For this review, take the finished solid that the model builds, in its own axes (mm). A direction names the side the tool comes from. Coordinates: 2 decimals unless noted, no trailing zeros. Write each loop counter-clockwise with the first axis right and the second up, starting at its lowest first coordinate (ties: lowest second). Pieces come first, ordered by that corner, then holes.
```python
from build123d import *

# Parameters (mm, degrees)
F0_W      = 76.2
F0_H      = 76.2
F1_DEPTH  = 76.2
F4_DEPTH  = 76.2
F5_DEPTH  = 76.2
F8_DEPTH  = 76.2
F9_DEPTH  = 76.2
F11_DEPTH = 76.2
F13_DEPTH = 76.2
F14_DEPTH = 25.4
F15_DEPTH = 25.4
F16_DEPTH = 25.4
F17_DEPTH = 25.4
F18_DEPTH = 25.4
F19_DEPTH = 25.4
F20_DEPTH = 25.4
F21_DEPTH = 25.4
F22_DEPTH = 25.4


with BuildPart() as f1:
    # F0 (on Front) → F1 (new body)
    with BuildSketch(Plane.XZ):
        Rectangle(F0_W, F0_H)
    extrude(amount=F1_DEPTH)

    # F2 (on face) → F4 (join)
    with BuildSketch(Plane.XZ.offset(76.2)):
        with BuildLine():
            ThreePointArc((0, -38.1), (26.9407683632, -26.9407683632), (38.1, 0))
            ThreePointArc((38.1, 0), (26.9407683632, 26.9407683632), (0, 38.1))
            ThreePointArc((0, 38.1), (-26.9407683632, 26.9407683632), (-38.1, 0))
            ThreePointArc((-38.1, 0), (-26.9407683632, -26.9407683632), (0, -38.1))
        make_face()
    extrude(amount=-F4_DEPTH)

    # F3 (on face) → F5 (join)
    with BuildSketch(Plane.YZ.offset(38.1)):
        with BuildLine():
            ThreePointArc((-38.1, -38.1), (-11.1592316368, -26.9407683632), (0, 0))
            ThreePointArc((0, 0), (-11.1592316368, 26.9407683632), (-38.1, 38.1))
            ThreePointArc((-38.1, 38.1), (-65.0407683632, 26.9407683632), (-76.2, 0))
            ThreePointArc((-76.2, 0), (-65.0407683632, -26.9407683632), (-38.1, -38.1))
        make_face()
    extrude(amount=-F5_DEPTH)

    # F7 (on face) → F8 (join)
    with BuildSketch(Plane(origin=(0, 0, 0), x_dir=(-1, 0, 0), z_dir=(0, 1, 0))):
        with BuildLine():
            ThreePointArc((0, -38.1), (26.9407683632, -26.9407683632), (38.1, 0))
            ThreePointArc((38.1, 0), (26.9407683632, 26.9407683632), (0, 38.1))
            ThreePointArc((0, 38.1), (-26.9407683632, 26.9407683632), (-38.1, 0))
            ThreePointArc((-38.1, 0), (-26.9407683632, -26.9407683632), (0, -38.1))
        make_face()
    extrude(amount=-F8_DEPTH)



with BuildPart() as f9:
    # F6 (on face) → F9 (new body)
    with BuildSketch(Plane(origin=(-38.1, 0, 0), x_dir=(0, -1, 0), z_dir=(-1, 0, 0))):
        with BuildLine():
            ThreePointArc((38.1, -38.1), (65.0407683632, -26.9407683632), (76.2, 0))
            ThreePointArc((76.2, 0), (65.0407683632, 26.9407683632), (38.1, 38.1))
            ThreePointArc((38.1, 38.1), (11.1592316368, 26.9407683632), (0, 0))
            ThreePointArc((0, 0), (11.1592316368, -26.9407683632), (38.1, -38.1))
        make_face()
    extrude(amount=-F9_DEPTH)


with BuildPart() as f1_1:
    add(f1.part)

    add(f9.part)  # F11 merges F9
    # F10 (on face) → F11 (join)
    with BuildSketch(Plane.XY.offset(38.1)):
        with BuildLine():
            ThreePointArc((0, -76.2), (26.9407683632, -65.0407683632), (38.1, -38.1))
            ThreePointArc((38.1, -38.1), (26.9407683839, -11.1592316575), (5.86e-08, 0))
            ThreePointArc((5.86e-08, 0), (-26.9407683425, -11.1592316161), (-38.1, -38.1))
            ThreePointArc((-38.1, -38.1), (-26.9407683632, -65.0407683632), (0, -76.2))
        make_face()
    extrude(amount=-F11_DEPTH)

    # F12 (on face) → F13 (join)
    with BuildSketch(Plane(origin=(0, 0, -38.1), x_dir=(1, 0, 0), z_dir=(0, 0, -1))):
        with BuildLine():
            ThreePointArc((8.43e-08, 0), (26.940768393, 11.1592316666), (38.1, 38.1))
            ThreePointArc((38.1, 38.1), (26.9407683632, 65.0407683632), (0, 76.2))
            ThreePointArc((0, 76.2), (-26.9407683632, 65.0407683632), (-38.1, 38.1))
            ThreePointArc((-38.1, 38.1), (-26.9407683334, 11.159231607), (8.43e-08, 0))
        make_face()
    extrude(amount=-F13_DEPTH)

    # F2 (on face) → F14 (cut)
    with BuildSketch(Plane.XZ.offset(76.2)):
        with BuildLine():
            ThreePointArc((0, 38.1), (26.9407683632, 26.9407683632), (38.1, 0))
            Line((38.1, 0), (38.1, 38.1))
            Line((38.1, 38.1), (0, 38.1))
        make_face()
    extrude(amount=-F14_DEPTH, mode=Mode.SUBTRACT)

    # F2 (on face) → F15 (cut)
    with BuildSketch(Plane.XZ.offset(76.2)):
        with BuildLine():
            ThreePointArc((-38.1, 0), (-26.9407683632, 26.9407683632), (0, 38.1))
            Line((0, 38.1), (-38.1, 38.1))
            Line((-38.1, 38.1), (-38.1, 0))
        make_face()
    extrude(amount=-F15_DEPTH, mode=Mode.SUBTRACT)

    # F2 (on face) → F16 (cut)
    with BuildSketch(Plane.XZ.offset(76.2)):
        with BuildLine():
            Line((38.1, -38.1), (38.1, 0))
            ThreePointArc((38.1, 0), (26.9407683632, -26.9407683632), (0, -38.1))
            Line((0, -38.1), (38.1, -38.1))
        make_face()
        with BuildLine():
            Line((-38.1, -38.1), (0, -38.1))
            ThreePointArc((0, -38.1), (-26.9407683632, -26.9407683632), (-38.1, 0))
            Line((-38.1, 0), (-38.1, -38.1))
        make_face()
    extrude(amount=-F16_DEPTH, mode=Mode.SUBTRACT)

    # F3 (on face) → F17 (cut)
    with BuildSketch(Plane.YZ.offset(38.1)):
        with BuildLine():
            ThreePointArc((-76.2, 0), (-65.0407683632, 26.9407683632), (-38.1, 38.1))
            Line((-38.1, 38.1), (-76.2, 38.1))
            Line((-76.2, 38.1), (-76.2, 0))
        make_face()
    extrude(amount=-F17_DEPTH, mode=Mode.SUBTRACT)

    # F3 (on face) → F18 (cut)
    with BuildSketch(Plane.YZ.offset(38.1)):
        with BuildLine():
            ThreePointArc((-38.1, 38.1), (-11.1592316368, 26.9407683632), (0, 0))
            Line((0, 0), (0, 38.1))
            Line((0, 38.1), (-38.1, 38.1))
        make_face()
        with BuildLine():
            Line((0, -38.1), (0, 0))
            ThreePointArc((0, 0), (-11.1592316368, -26.9407683632), (-38.1, -38.1))
            Line((-38.1, -38.1), (0, -38.1))
        make_face()
        with BuildLine():
            Line((-76.2, -38.1), (-38.1, -38.1))
            ThreePointArc((-38.1, -38.1), (-65.0407683632, -26.9407683632), (-76.2, 0))
            Line((-76.2, 0), (-76.2, -38.1))
        make_face()
        with BuildLine():
            ThreePointArc((-76.2, 0), (-65.0407683632, 26.9407683632), (-38.1, 38.1))
            Line((-38.1, 38.1), (-76.2, 38.1))
            Line((-76.2, 38.1), (-76.2, 0))
        make_face()
    extrude(amount=-F18_DEPTH, mode=Mode.SUBTRACT)

    # F6 (on face) → F19 (cut)
    with BuildSketch(Plane(origin=(-38.1, 0, 0), x_dir=(0, -1, 0), z_dir=(-1, 0, 0))):
        with BuildLine():
            ThreePointArc((0, 0), (11.1592316368, 26.9407683632), (38.1, 38.1))
            Line((38.1, 38.1), (0, 38.1))
            Line((0, 38.1), (0, 0))
        make_face()
        with BuildLine():
            ThreePointArc((38.1, 38.1), (65.0407683632, 26.9407683632), (76.2, 0))
            Line((76.2, 0), (76.2, 38.1))
            Line((76.2, 38.1), (38.1, 38.1))
        make_face()
        with BuildLine():
            Line((76.2, -38.1), (76.2, 0))
            ThreePointArc((76.2, 0), (65.0407683632, -26.9407683632), (38.1, -38.1))
            Line((38.1, -38.1), (76.2, -38.1))
        make_face()
        with BuildLine():
            Line((0, -38.1), (38.1, -38.1))
            ThreePointArc((38.1, -38.1), (11.1592316368, -26.9407683632), (0, 0))
            Line((0, 0), (0, -38.1))
        make_face()
    extrude(amount=-F19_DEPTH, mode=Mode.SUBTRACT)

    # F7 (on face) → F20 (cut)
    with BuildSketch(Plane(origin=(0, 0, 0), x_dir=(-1, 0, 0), z_dir=(0, 1, 0))):
        with BuildLine():
            ThreePointArc((-38.1, 0), (-26.9407683632, 26.9407683632), (0, 38.1))
            Line((0, 38.1), (-38.1, 38.1))
            Line((-38.1, 38.1), (-38.1, 0))
        make_face()
        with BuildLine():
            ThreePointArc((0, 38.1), (26.9407683632, 26.9407683632), (38.1, 0))
            Line((38.1, 0), (38.1, 38.1))
            Line((38.1, 38.1), (0, 38.1))
        make_face()
        with BuildLine():
            Line((38.1, -38.1), (38.1, 0))
            ThreePointArc((38.1, 0), (26.9407683632, -26.9407683632), (0, -38.1))
            Line((0, -38.1), (38.1, -38.1))
        make_face()
        with BuildLine():
            Line((-38.1, -38.1), (0, -38.1))
            ThreePointArc((0, -38.1), (-26.9407683632, -26.9407683632), (-38.1, 0))
            Line((-38.1, 0), (-38.1, -38.1))
        make_face()
    extrude(amount=-F20_DEPTH, mode=Mode.SUBTRACT)

    # F10 (on face) → F21 (cut)
    with BuildSketch(Plane.XY.offset(38.1)):
        with BuildLine():
            ThreePointArc((5.86e-08, 0), (26.9407683839, -11.1592316575), (38.1, -38.1))
            Line((38.1, -38.1), (38.1, 0))
            Line((38.1, 0), (5.86e-08, 0))
        make_face()
        with BuildLine():
            Line((38.1, -76.2), (38.1, -38.1))
            ThreePointArc((38.1, -38.1), (26.9407683632, -65.0407683632), (0, -76.2))
            Line((0, -76.2), (38.1, -76.2))
        make_face()
        with BuildLine():
            Line((-38.1, -76.2), (0, -76.2))
            ThreePointArc((0, -76.2), (-26.9407683632, -65.0407683632), (-38.1, -38.1))
            Line((-38.1, -38.1), (-38.1, -76.2))
        make_face()
        with BuildLine():
            ThreePointArc((-38.1, -38.1), (-26.9407683425, -11.1592316161), (5.86e-08, 0))
            Line((5.86e-08, 0), (-38.1, 0))
            Line((-38.1, 0), (-38.1, -38.1))
        make_face()
    extrude(amount=-F21_DEPTH, mode=Mode.SUBTRACT)

    # F12 (on face) → F22 (cut)
    with BuildSketch(Plane(origin=(0, 0, -38.1), x_dir=(1, 0, 0), z_dir=(0, 0, -1))):
        with BuildLine():
            Line((-38.1, 0), (8.43e-08, 0))
            ThreePointArc((8.43e-08, 0), (-26.9407683334, 11.159231607), (-38.1, 38.1))
            Line((-38.1, 38.1), (-38.1, 0))
        make_face()
        with BuildLine():
            ThreePointArc((-38.1, 38.1), (-26.9407683632, 65.0407683632), (0, 76.2))
            Line((0, 76.2), (-38.1, 76.2))
            Line((-38.1, 76.2), (-38.1, 38.1))
        make_face()
        with BuildLine():
            ThreePointArc((0, 76.2), (26.9407683632, 65.0407683632), (38.1, 38.1))
            Line((38.1, 38.1), (38.1, 76.2))
            Line((38.1, 76.2), (0, 76.2))
        make_face()
        with BuildLine():
            Line((38.1, 0), (38.1, 38.1))
            ThreePointArc((38.1, 38.1), (26.940768393, 11.1592316666), (8.43e-08, 0))
            Line((8.43e-08, 0), (38.1, 0))
        make_face()
    extrude(amount=-F22_DEPTH, mode=Mode.SUBTRACT)


solid = f1_1.part
```
1) Tool access review of faces 1 (the face through (-30, -68, -12.7)), 2 (the face through (-30, -8, 12.7)), 3 (the face through (12.7, -76, 10)), 4 (the face through (12.7, -1, 10)): name each direction out of +Z, -Z, +X, -X, +Y, -Y from which nothing blocks a thin tool from reaching the whole face with its end or side.
2) Consider section D-D (y = -53). Give the boundary of the cut face in (x, z).
3) Consider section A-A (y = -68). Give the boundary of the cut face in (x, z).
4) Clearance check with flat-ended pins moving along their axes: P1, Ø2.5, axis at x = 3.5, z = -37, coming from the -Y side; P2, Ø2.5, axis at x = 5, y = -1.5, coming from the +Z side (3 decimals); P3, Ø1.1, axis at x = 37, z = -6.5, coming from the -Y side; P4, Ø12, axis at x = -17, z = -6.5, coming from the +Y side. State where each tip first meets the part, or that it passes through.
5) For L1, parallel to X at y = -10, z = 30; L2, parallel to Y at x = -32.5, z = 33.5; L3, parallel to X at y = -69, z = -1, list the stretches that pass through material, from the lowest coordinate up.
6) Consider section B-B (x = -28). Give the boundary of the cut face in (y, z).
7) Consider section C-C (z = 14). Give the boundary of the cut face in (x, y).
Results:
1. face 1: -Z, -X, -Y
1. face 2: +Z, -X, +Y
1. face 3: +Z, +X, -Y
1. face 4: +Z, +X, +Y
2. outline: (-35.92, -12.7) - (-35.07, -12.7) - (-35.07, -14.9) arc R38.1 ccw to (-14.9, -35.07) - (-12.7, -35.07) - (-12.7, -35.92) arc R38.1 ccw to (12.7, -35.92) - (12.7, -35.07) - (14.9, -35.07) arc R38.1 ccw to (35.07, -14.9) - (35.07, -12.7) - (35.92, -12.7) arc R38.1 ccw to (35.92, 12.7) - (35.07, 12.7) - (35.07, 14.9) arc R38.1 ccw to (14.9, 35.07) - (12.7, 35.07) - (12.7, 35.92) arc R38.1 ccw to (-12.7, 35.92) - (-12.7, 35.07) - (-14.9, 35.07) arc R38.1 ccw to (-35.07, 14.9) - (-35.07, 12.7) - (-35.92, 12.7) arc R38.1 ccw to start
3. outline: (-35.92, -12.7) - (-23.61, -12.7) - (-23.61, -23.61) - (-12.7, -23.61) - (-12.7, -35.92) arc R38.1 ccw to (12.7, -35.92) - (12.7, -23.61) - (23.61, -23.61) - (23.61, -12.7) - (35.92, -12.7) arc R38.1 ccw to (35.92, 12.7) - (23.61, 12.7) - (23.61, 23.61) - (12.7, 23.61) - (12.7, 35.92) arc R38.1 ccw to (-12.7, 35.92) - (-12.7, 23.61) - (-23.61, 23.61) - (-23.61, 12.7) - (-35.92, 12.7) arc R38.1 ccw to start
4. P1: stops at y = -76.13
4. P2: stops at z = 37.915
4. P3: stops at y = -75.73
4. P4: stops at y = 0
5. L1: x = -12.7 to 12.7
5. L2: y = -50.8 to -25.4
5. L3: x = -38.09 to 38.09
6. outline: (-74.02, -12.7) - (-63.94, -12.7) - (-63.94, -25.84) - (-50.8, -25.84) - (-50.8, -35.92) arc R38.1 ccw to (-25.4, -35.92) - (-25.4, -25.84) - (-12.26, -25.84) - (-12.26, -12.7) - (-2.18, -12.7) arc R38.1 ccw to (-2.18, 12.7) - (-12.26, 12.7) - (-12.26, 25.84) - (-25.4, 25.84) - (-25.4, 35.92) arc R38.1 ccw to (-50.8, 35.92) - (-50.8, 25.84) - (-63.94, 25.84) - (-63.94, 12.7) - (-74.02, 12.7) arc R38.1 ccw to start
7. outline: (-35.92, -50.8) - (-35.43, -50.8) - (-35.43, -52.1) arc R38.1 ccw to (-14, -73.53) - (-12.7, -73.53) - (-12.7, -74.02) arc R38.1 ccw to (12.7, -74.02) - (12.7, -73.53) - (14, -73.53) arc R38.1 ccw to (35.43, -52.1) - (35.43, -50.8) - (35.92, -50.8) arc R38.1 ccw to (35.92, -25.4) - (35.43, -25.4) - (35.43, -24.1) arc R38.1 ccw to (14, -2.67) - (12.7, -2.67) - (12.7, -2.18) arc R38.1 ccw to (-12.7, -2.18) - (-12.7, -2.67) - (-14, -2.67) arc R38.1 ccw to (-35.43, -24.1) - (-35.43, -25.4) - (-35.92, -25.4) arc R38.1 ccw to start
